CAD build for the part. Positions are in the model's coordinates, mm. A direction names the side the tool comes from. Give positions to 0.01 mm unless a question says otherwise; leave off trailing zeros. Write each loop counter-clockwise with the first axis right and the second up, starting at its lowest first coordinate (ties: lowest second). Pieces come first, ordered by that corner, then holes. Notation, with made-up numbers: (39, 84.25) - (97, 84.25) arc R20 ccw to (97, 105.25) - close; hole circle Ø9 at (60.5, 45). An arc over 180 degrees is marked (long way). Put each result on its own line as item: value. Start each with the question number.
1. Cut at A-A on y = 0. List the corners of the cut face in (x, z), and give its area (3 significant figures).
2. Tool access for faces 1 (the cylindrical face through (-20.37, 9.34, 7.52)), 2 (the flat face through (-14.467, 23.37, 1.878)): list every direction of +Z, -Z, +X, -X, +Y, -Y with a clear straight run to the whole face (end or side of a thin tool).
3. Wall check: line 1 (Y direction, x = -9.5, z = 7.75); line 2 (X direction, y = 0, z = 6.75); line 3 (Y direction, x = -17.5, z = 4). Give the ranges that are in metal, low to high.
4. Mould opens along X. For faces 3 (the flat face through (-11, 0, 6.35)), 4 (the cylindrical face through (19.004, 0.108, 6.796)), 5 (the cylindrical face through (22.9, 0.1, 3.2)), 6 (the cylindrical face through (0.76, 16.464, 7.665)) say: +X half, -X half, draft (parallel to the pull), parting line (faces both ways), or undercut.
5. Cut at B-B on z = 2. Give the number of separate pieces and of enclosed holes in the cut face, and give its area (3 significant figures).
6. Drop flat-ended pins along their axis: pin 1 (1.5 mm diameter, centred on y = 8.5, z = 1, fed in from +X); pin 2 (2 mm diameter, centred on x = -0.5, y = 18.5, fed in from -Z); pin 3 (1.5 mm diameter, centred on y = -24, z = 4.5, fed in from +X). Give the stop position or say it passes through.
from build123d import *

# Parameters (mm, degrees)
BOSS_EXTRUDE1_DEPTH                               = 8.73125
SKETCH2_R                                         = 101.6
SKETCH2_R_2                                       = 76.2
CUT_EXTRUDE1_DEPTH                                = 58.485257961
FILLET1_R                                         = 9.525
CSK_FOR_8_FLAT_HEAD_MACHINE_SCREW_100_D           = 4.9149
CSK_FOR_8_FLAT_HEAD_MACHINE_SCREW_100_CSINK_D     = 8.4328
CSK_FOR_8_FLAT_HEAD_MACHINE_SCREW_100_CSINK_ANGLE = 100
CUT_EXTRUDE2_START                                = -6.35
CUT_EXTRUDE2_DEPTH                                = 6.35
CUT_EXTRUDE3_DEPTH                                = 3.81
SKETCH7_R                                         = 1.397
CUT_EXTRUDE4_DEPTH                                = 3.175
HOLE1_AT_2_COUNT                                  = 2
HOLE1_AT_2_PITCH                                  = 9.3599
HOLE1_AT_3_COUNT                                  = 2
HOLE1_AT_3_PITCH                                  = 38.818175673
HOLE1_AT_4_COUNT                                  = 2
HOLE1_AT_4_PITCH                                  = 40.17317123
F_2_CLEARANCE_HOLE1_D                             = 2.7051
F_2_CLEARANCE_HOLE1_DEPTH                         = 4.7625


with BuildPart() as part:
    # Sketch1 → Boss-Extrude1 (new body)
    with BuildSketch(Plane.XY):
        Polygon((33.299680929, 0), (-33.299680929, 46.0375), (-33.299680929, -46.0375), align=None)
    extrude(amount=BOSS_EXTRUDE1_DEPTH)

    # Sketch2 → Cut-Extrude1 (cut, through all)
    with BuildSketch(Plane.XY.offset(8.73125)):
        with Locations((42.900319071, 0)):
            Circle(SKETCH2_R)
        with Locations((42.900319071, 0)):
            Circle(SKETCH2_R_2, mode=Mode.SUBTRACT)
    extrude(amount=-CUT_EXTRUDE1_DEPTH, mode=Mode.SUBTRACT)

    # Fillet1
    fillet1_edges = [part.edges().sort_by_distance(p)[0] for p in [
        (-22.72460624, -38.727369881, 4.365625),
        (-22.72460624, 38.727369881, 4.365625),
        (33.299680929, 0, 4.365625),
    ]]
    fillet(fillet1_edges, radius=FILLET1_R)

    # CSK for #8 Flat Head Machine Screw (100)1 (through all)
    with Locations(Plane.XY.offset(8.73125)):
        with Locations((-19.063658953, -24.617494846), (-19.063658953, 24.617494846), (16.54881886, 0)):
            CounterSinkHole(CSK_FOR_8_FLAT_HEAD_MACHINE_SCREW_100_D / 2, CSK_FOR_8_FLAT_HEAD_MACHINE_SCREW_100_CSINK_D / 2, counter_sink_angle=CSK_FOR_8_FLAT_HEAD_MACHINE_SCREW_100_CSINK_ANGLE)

    # Sketch5 → Cut-Extrude2 (cut)
    with BuildSketch(Plane(origin=(0, 0, 0), x_dir=(-1, 0, 0), z_dir=(0, 0, -1)).offset(CUT_EXTRUDE2_START)):
        with BuildLine():
            Line((30.823542048, 19.267389595), (-18.192319797, 6.133628997))
            ThreePointArc((-18.192319797, 6.133628997), (-22.89881886, 0), (-18.192319797, -6.133628997))
            Line((-18.192319797, -6.133628997), (30.823542048, -19.267389595))
            ThreePointArc((30.823542048, -19.267389595), (33.299680929, 0), (30.823542048, 19.267389595))
        make_face()
    extrude(amount=CUT_EXTRUDE2_DEPTH, mode=Mode.SUBTRACT)

    # Sketch6 → Cut-Extrude3 (cut)
    with BuildSketch(Plane(origin=(0, 0, 0), x_dir=(-1, 0, 0), z_dir=(0, 0, -1))):
        Polygon((16.588726313, -15.453182214), (-4.265612277, -9.86527903), (-8.867414899, -27.039440222), (11.986923691, -32.627343405), align=None)
        Polygon((11.986923691, 32.627343405), (-8.867414899, 27.039440222), (-4.265612277, 9.86527903), (16.588726313, 15.453182214), align=None)
    extrude(amount=-CUT_EXTRUDE3_DEPTH, mode=Mode.SUBTRACT)

    # Sketch7 → Cut-Extrude4 (cut)
    with BuildSketch(Plane(origin=(0, 0, 6.35), x_dir=(-1, 0, 0), z_dir=(0, 0, -1))):
        with Locations((21.479680921, -10.189705806)):
            Circle(SKETCH7_R)
        with Locations((21.479680921, 10.189705806)):
            Circle(SKETCH7_R)
    extrude(amount=-CUT_EXTRUDE4_DEPTH, mode=Mode.SUBTRACT)

    # Sketch9 → Hole1 (revolve, cut)
    with BuildSketch(Plane(origin=(-8.904685942, -20.086585615, 3.81), x_dir=(0, 1, 0), z_dir=(1, 0, 0))):
        Polygon((0, 0), (0, 2.921), (1.4986, 2.921), (1.6383, 0), align=None)
    hole1 = revolve(axis=Axis((-8.904685942, -20.086585615, 113.81), (0, 0, -1)), mode=Mode.SUBTRACT)

    # Hole1 at 2: Hole1 ×2
    with Locations(*[Vector(0.9659258262890683, 0.25881904510252096, 0) * (i * HOLE1_AT_2_PITCH) for i in range(1, HOLE1_AT_2_COUNT)]):
        add(hole1, mode=Mode.SUBTRACT)

    # Hole1 at 3: Hole1 ×2
    with Locations(*[Vector(0.23290556510295454, 0.9724993561664057, 0) * (i * HOLE1_AT_3_PITCH) for i in range(1, HOLE1_AT_3_COUNT)]):
        add(hole1, mode=Mode.SUBTRACT)

    # Hole1 at 4: Hole1 ×2
    with Locations(*[(0, i * HOLE1_AT_4_PITCH, 0) for i in range(1, HOLE1_AT_4_COUNT)]):
        add(hole1, mode=Mode.SUBTRACT)

    # #2 Clearance Hole1
    with Locations(Plane(origin=(0, 0, 3.81), x_dir=(-1, 0, 0), z_dir=(0, 0, -1))):
        with Locations((8.904685942, -20.086585615), (-0.136283199, -17.664065235), (-0.136283199, 17.664065235), (8.904685942, 20.086585615)):
            Hole(F_2_CLEARANCE_HOLE1_D / 2, depth=F_2_CLEARANCE_HOLE1_DEPTH)


solid = part.part
Report:
1. outline: (-33.3, 6.35) - (14.09, 6.35) - (14.09, 7.26) - (12.33, 8.73) - (-33.3, 8.73) - close; (19.01, 6.35) - (22.9, 6.35) - (22.9, 0) - (26.07, 0) - (26.07, 8.73) - (20.77, 8.73) - (19.01, 7.26) - close
1. area: 147 mm²
2. face 1: +Z, -Z
2. face 2: -Z
3. line 1: y = -29.59 to -21.3, -18.87 to 18.87, 21.3 to 29.59
3. line 2: x = -33.3 to 14.09, 19.01 to 26.07
3. line 3: y = -34.01 to -26.51, -22.72 to -15.7, 15.7 to 22.72, 26.51 to 34.01
4. face 3: draft
4. face 4: undercut
4. face 5: -X half
4. face 6: undercut
5. separate pieces: 3
5. enclosed holes: 2
5. area: 682 mm²
6. pin 1: stops at x = 22.09
6. pin 2: stops at z = 3.81
6. pin 3: stops at x = -0.33
